Autodesk Inventor part; units mm, degrees
ref_plane "YZ Plane" through (0, 0, 0) normal (1, 0, 0) x (0, 1, 0)
ref_plane "XZ Plane" through (0, 0, 0) normal (0, 1, 0) x (-1, 0, 0)
ref_plane "XY Plane" through (0, 0, 0) normal (0, 0, 1) x (1, 0, 0)
sketch "Sketch1" plane through (0, 0, 0) normal (0, 1, 0) x (-1, 0, 0)
  line L0 (50, 0) -> (0, 0)
  line L1 (50, -10) -> (50, 0)
  line L2 (12, -10) -> (50, -10)
  line L3 (12, -22) -> (12, -10)
  line L4 (0, -22) -> (12, -22)
  line L5 (0, 0) -> (0, -22)
extrude "Extrusion1" add sketch "Sketch1" along normal blind 1.27
sketch "Sketch2" plane through (0, 1.27, 0) normal (0, 1, 0) x (1, 0, 0)
  point P0 (-6, 17)
hole "Hole1" at (-6, 1.27, -17) direction (0, -1, 0) diameter 4 depth 1.27
properties part number "Y-axis X-axis Flag" material "Nylon 6/6"
Work out the finished part from the listing and answer in its coordinate system (mm). A direction names the side the tool comes from. Give positions to 0.01 mm unless a question says otherwise; leave off trailing zeros. Order: outer loops, then holes, each group sorted by start corner. A loop starts at its lowest first (then second) coordinate and runs counter-clockwise, first axis right, second up. Notation, with made-up numbers: (48.5, 41.5) -> (91.5, 41.5) arc R11 cw to (91.5, 49.5) -> close; hole circle Ø11 at (-3.5, -32.75). An arc over 180 degrees is marked (long way). Answer as CSV lines item,"result". Start each with the question number.
(1) Section C-C, the plane y = 0.9 is taken. Write down the section's boundary in (x, z).
(2) Section A-A, the plane z = -17 is taken. Write down the section's boundary in (x, y), plus the area to 3 significant figures.
(3) Section D-D, the plane z = -19.75 is taken. Write down the section's boundary in (x, y).
(4) Consider line 1 along X through (y, z) = (1.05, -17); line 2 along Z through (x, y) = (-6, 0.6); line 3 along Z through (x, y) = (-36.5, 0.85). Determine where each line is inside the solid, lowest interval first.
(5) Which of the six approach directions +Z, -Z, +X, -X, +Y, -Y give full straight-line access (tool end or side, diameter ignored) to faces 1 (the flat face through (-19, 0, -6)), 2 (the flat face through (-12, 1, -16))?
(6) For a pull along Z with two mould halves and no side action, classify faces 3 (the flat face through (-25, 1, 0)), 4 (the flat face through (-19, 1.27, -6)), 5 (the cylindrical face through (-7.352, 0.626, -18.474)) as released by +Z, released by -Z, zero draft, split by the parting line, or undercut.
(7) Section B-B, the plane x = -6 is taken. Write down the section's boundary in (y, z).
Entries:
1,outline,"(-50, -10) -> (-12, -10) -> (-12, -22) -> (0, -22) -> (0, 0) -> (-50, 0) -> close; hole circle Ø4 at (-6, -17)"
2,outline,"(-12, 0) -> (-8, 0) -> (-8, 1.27) -> (-12, 1.27) -> close; (-4, 0) -> (0, 0) -> (0, 1.27) -> (-4, 1.27) -> close"
2,area,"10.2 mm²"
3,outline,"(-12, 0) -> (0, 0) -> (0, 1.27) -> (-12, 1.27) -> close"
4,line 1,"-12 to -8, -4 to 0"
4,line 2,"-22 to -19, -15 to 0"
4,line 3,"-10 to 0"
5,face 1,"+Z, -Z, +X, -X, -Y"
5,face 2,"-Z, -X, +Y, -Y"
6,face 3,"released by +Z"
6,face 4,"zero draft"
6,face 5,"undercut"
7,outline,"(0, -22) -> (1.27, -22) -> (1.27, -19) -> (0, -19) -> close; (0, -15) -> (1.27, -15) -> (1.27, 0) -> (0, 0) -> close"
